Geometry: see drawing. Coordinates: mm, zero at the bounding-box minimum. A direction names the side the tool comes from. Round coordinates to 2 decimals unless told otherwise and drop trailing zeros. Order: outer loops, then holes, each group sorted by start corner. A loop starts at its lowest first (then second) coordinate and runs counter-clockwise, first axis right, second up. Notation, with made-up numbers: (76, -13) -> (130, -13) arc R26 cw to (130, 20) -> close; hole circle Ø10 at (21, -35). An arc over 180 degrees is marked (long way). Write item = value, one per line. Start each with the question number.
(1) Draft query along X for the marked faces 1, 2, 3 and 4. Return one class per face: released by +X, released by -X, zero draft, split by the parting line, or undercut.
(2) Cut plane B-B on x = 54. Return the cut outline in (y, z), then the cut area to 3 significant figures.
(3) Ray query, line 1 (X direction, y = 5.25, z = 23.5) (1 decimal); line 2 (Z direction, x = 54, y = 0.7); line 3 (X direction, y = 1, z = 6.25) (1 decimal). Return the intervals inside material, ascending.
(4) Reachability of the marked faces 5 and 6 from +Z, -Z, +X, -X, +Y, -Y: full face, straight path, thin tool, end or side. Return the list, or none.
(5) Cut plane C-C on z = 16. Return the cut outline in (x, y) (1 decimal).
(6) Contact query for flat-ended pins moving along their axis: pin 1 Ø6.5 at (x, y) = (53, 6) entering from -Z; pin 2 Ø1 at (x, z) = (48, 18) entering from +Y; pin 3 Ø9 at (x, z) = (53.5, 12.5) entering from +Y. Output: stop coordinate, or through.
(7) Cut plane D-D on y = 3.25. Return the cut outline in (x, z) (1 decimal).
(8) Cut plane A-A on z = 5.5. Give the number of separate pieces and of enclosed holes in the cut face, then the cut area to 3 significant figures.
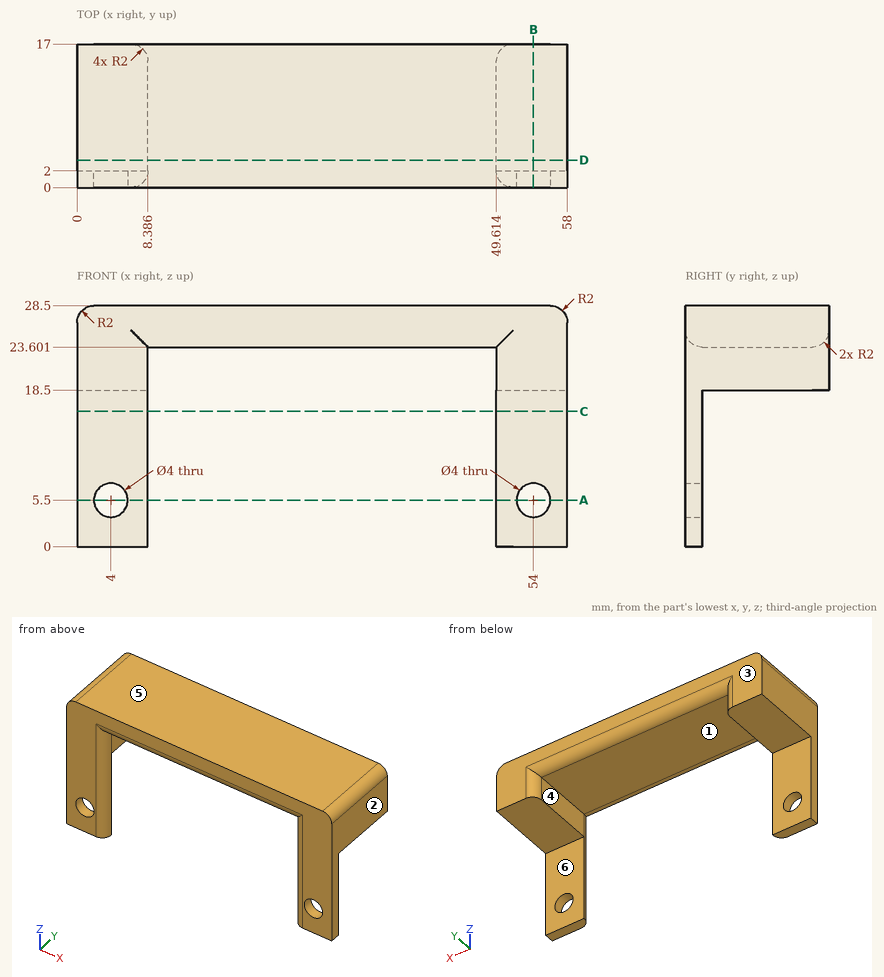
Evaluation:
q1.face_1 = undercut
q1.face_2 = released by +X
q1.face_3 = zero draft
q1.face_4 = undercut
q2.outline = (0, 0) -> (2, 0) -> (2, 3.5) -> (0, 3.5) -> close; (0, 7.5) -> (2, 7.5) -> (2, 18.5) -> (17, 18.5) -> (17, 28.5) -> (0, 28.5) -> close
q2.area = 199 mm^2
q3.line_1 = 0 to 8.4, 49.6 to 58
q3.line_2 = 0 to 3.5, 7.5 to 28.5
q3.line_3 = 0 to 2.1, 5.9 to 8.1, 49.9 to 52.1, 55.9 to 58
q4.face_5 = +Z, +X, -X, +Y, -Y
q4.face_6 = -Z, +X, -X, +Y
q5.outline = (0, 0) -> (6.4, 0) arc R2 ccw to (8.4, 2) -> (0, 2) -> close; (49.6, 2) arc R2 ccw to (51.6, 0) -> (58, 0) -> (58, 2) -> close
q6.pin_1 = 18.5
q6.pin_2 = through
q6.pin_3 = 2
q7.outline = (0, 18.5) -> (8.4, 18.5) -> (8.4, 23.6) -> (49.6, 23.6) -> (49.6, 18.5) -> (58, 18.5) -> (58, 26.5) arc R2 ccw to (56, 28.5) -> (2, 28.5) arc R2 ccw to (0, 26.5) -> close
q8.separate_pieces = 4
q8.enclosed_holes = 0
q8.area = 15.8 mm^2
